Autodesk Fusion 360 part; units mm, degrees
sketch "Sketch1" plane through (0, 0, 0) normal (0, 0, 1) x (1, 0, 0)
  circle A0 centre (0, 0) radius 8
  line L0 (0, 16) -> (36, 16)
  line L1 (36, 16) -> (36, -16)
  line L2 (36, -16) -> (0, -16)
  arc A1 (0, 16) -> (0, -16) centre (0, 0) ccw
  dimension "d1" = 16
  dimension "d2" = 32
  dimension "d3" = 36
  dimension "d4" = 32
extrude "Extrude1" add sketch "Sketch1" along normal blind 11
sketch "Sketch2" plane through (0, 0, 11) normal (0, 0, 1) x (-1, 0, 0)
  circle A0 centre (0, 0) radius 8
  line L0 (-36, -16) -> (0, -16)
  arc A1 (0, -16) -> (0, 16) centre (0, 0) ccw
  line L1 (0, 16) -> (-36, 16)
  line L2 (-36, 16) -> (-36, -16)
  line L3 (-36, -16) -> (-25, -16)
  line L4 (-25, -16) -> (-25, 16)
  line L5 (-25, 16) -> (-36, 16)
  line L6 (-36, 16) -> (-36, -16)
  dimension "d7" = 11
  dimension "d8" = 32
extrude "Extrude2" add sketch "Sketch2" along normal blind 18 contours L0 L1 L2 L3 L4 L5 L6
sketch "Sketch3" plane through (0, 0, 29) normal (0, 0, 1) x (-1, 0, 0)
  line L0 (-36, 16) -> (-36, -16)
  line L1 (-36, -16) -> (-25, -16)
  line L2 (-25, -16) -> (-25, 16)
  line L3 (-25, 16) -> (-36, 16)
  line L4 (-36, -16) -> (0, -16)
  line L5 (0, -16) -> (0, 16)
  line L6 (0, 16) -> (-36, 16)
  line L7 (-36, 16) -> (-36, -16)
  circle A0 centre (0, 0) radius 8
  circle A1 centre (0, 0) radius 16
  dimension "d11" = 36
  dimension "d12" = 32
  dimension "d13" = 16
  dimension "d14" = 32
extrude "Extrude3" add sketch "Sketch3" along normal blind 11 contours L0 L1 L2 L3 L4 L6 L7 | L2 L4 L6 A1 | L5 A0 A1 | L5 A0 A1
sketch "Sketch4" plane through (36, 0, 0) normal (1, 0, 0) x (0, 1, 0)
  line L0 (-16, 0) -> (16, 0)
  line L1 (16, 0) -> (16, 40)
  line L2 (16, 40) -> (-16, 40)
  line L3 (-16, 40) -> (-16, 0)
  line L4 (16, 0) -> (16, 20)
  line L5 (16, 20) -> (0, 20)
  circle A0 centre (0, 20) radius 9
  dimension "d17" = 20
  dimension "d18" = 16
  dimension "d19" = 18
extrude "Extrude4" add sketch "Sketch4" along normal blind 32 contours A0
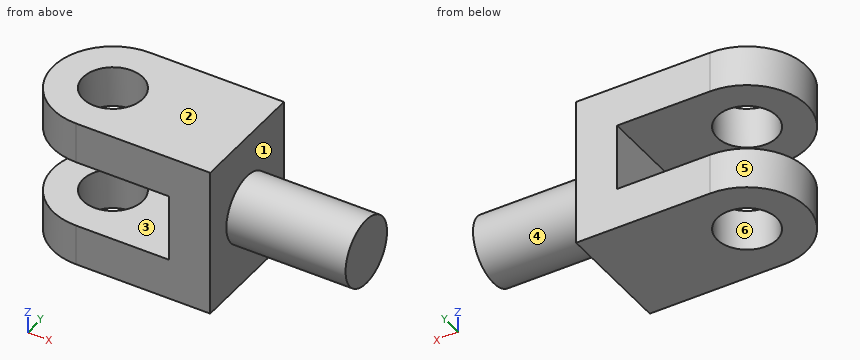
The model under review builds one solid part; all positions refer to its coordinate system, in mm. Face numbers are marked on the shaded views. A direction names the side the tool comes from. Give positions to 0.01 mm unless a question says otherwise; leave off trailing zeros. Order: outer loops, then holes, each group sorted by start corner. A loop starts at its lowest first (then second) coordinate and runs counter-clockwise, first axis right, second up. Notation, with made-up numbers: M 85,24 L 121,24 A35 cw 121,63 Z; hole C 76,-10 d7. An arc over 180 degrees is marked long. One line per question, with ' | ' between items. Start each with the question number.
1) Consider section C-C, the plane y = 0. Give the boundary of the cut face in (x, z).
2) For the marked faces 1, 2 and 3, list the 3-axis set-ups (+Z, -Z, +X, -X, +Y, -Y) from which the entire face can be reached by the end or side of a thin tool; tool diameter is ignored.
3) Mouldability with a two-part tool opening along X and no side actions: class the marked faces 4, 5 and 6 as pulls with the +X half, pulls with the -X half, needs draft (parallel to the pull), parting line crosses it, or undercut.
4) Wall thickness on L1, parallel to Y at x = 0, z = 35.25; L2, parallel to X at y = 0, z = 37; L3, parallel to Z at x = 24, y = 8.5: over which ranges is each line inside the solid? List them lowest first. Write a range as from..to.
5) Consider section A-A, the plane z = 9. Give the boundary of the cut face in (x, y).
6) Clearance check with flat-ended pins moving along their axes: P1, Ø6, axis at x = 48, z = 21, coming from the -Y side; P2, Ø3, axis at y = -7, z = 21, coming from the -X side; P3, Ø4, axis at x = 45.5, y = -12.5, coming from the -Z side; P4, Ø6, axis at y = 5, z = 9.5, coming from the -X side. State where each tip first meets the part, or that it passes through.
7) Consider section D-D, the plane z = 20. Give the boundary of the cut face in (x, y), then the cut area to 3 significant figures.
8) Consider section B-B, the plane x = 17. Give the boundary of the cut face in (y, z).
Found:
1) outline: M -16,0 L -8,0 L -8,11 L -16,11 Z; M -16,29 L -8,29 L -8,40 L -16,40 Z; M 8,0 L 36,0 L 36,11 L 68,11 L 68,29 L 36,29 L 36,40 L 8,40 L 8,29 L 25,29 L 25,11 L 8,11 Z
2) face 1: +X | face 2: +Z, +X, -X, +Y, -Y | face 3: -X, +Y, -Y
3) face 4: needs draft | face 5: pulls with the -X half | face 6: undercut
4) L1: y = -16..-8, 8..16 | L2: x = -16..-8, 8..36 | L3: z = 0..11, 29..40
5) outline: M 0,-16 L 36,-16 L 36,16 L 0,16 A16 ccw Z; hole C 0,0 d16
6) P1: stops at y = -9 | P2: stops at x = 25 | P3: passes through | P4: stops at x = -15.87
7) outline: M 25,-16 L 36,-16 L 36,-9 L 68,-9 L 68,9 L 36,9 L 36,16 L 25,16 Z | area: 928 mm²
8) outline: M -16,0 L 16,0 L 16,11 L -16,11 Z; M -16,29 L 16,29 L 16,40 L -16,40 Z
